from build123d import *

# Parameters (mm, degrees)
CUT_EXTRUDE1_DEPTH      = 874.621652083
CUT_EXTRUDE1_DEPTH_BACK = 874.621652083
SKETCH6_R               = 38.1
SKETCH9_W               = 1605.930086896
SKETCH9_H               = 1331.723127606
CUT_EXTRUDE8_DEPTH      = 762.168569892


with BuildPart() as part:
    # Sketch4 → Revolve3 (revolve)
    with BuildSketch(Plane.XY, mode=Mode.PRIVATE) as revolve3_sk:
        with BuildLine():
            Line((25.4, 650.00817936), (25.4, 83.643188795))
            ThreePointArc((25.4, 83.643188795), (205.276173143, 67.197534451), (381, 25.4))
            Line((381, 25.4), (412.7373, 25.4))
            Line((412.7373, 25.4), (412.7373, 488.95))
            Line((412.7373, 488.95), (411.1498, 488.95))
            Line((411.1498, 488.95), (411.1498, 514.35))
            ThreePointArc((411.1498, 514.35), (404.683813004, 537.626492136), (387.141395745, 554.23575674))
            ThreePointArc((387.141395745, 554.23575674), (211.762891066, 622.866495309), (25.4, 650.00817936))
        make_face()
    revolve(revolve3_sk.sketch.rotate(Axis((0, 588.703209944, 0), (0, -1, 0)), 90), axis=Axis((0, 588.703209944, 0), (0, -1, 0)))

    # Sketch6 → Cut-Extrude1 (cut, two sides: drawn at the far end of the back side and taken through both)
    with BuildSketch(Plane(origin=(0, 0, 0), x_dir=(1, 0, 0), z_dir=(0, 1, 0)).offset(-CUT_EXTRUDE1_DEPTH_BACK)):
        with Locations(Location((143.684097937, 143.684097937, 0), (0, 0, 131.539783137))):
            Circle(SKETCH6_R)
        with Locations(Location((-85.876030786, 184.161742326, 0), (0, 0, 134.878306021))):
            Circle(SKETCH6_R)
        with Locations(Location((-85.876030786, -184.161742326, 0), (0, 0, 134.996806388))):
            Circle(SKETCH6_R)
        with Locations(Location((143.684097937, -143.684097937, 0), (0, 0, 135))):
            Circle(SKETCH6_R)
    extrude(amount=CUT_EXTRUDE1_DEPTH + CUT_EXTRUDE1_DEPTH_BACK, mode=Mode.SUBTRACT)

    # Sketch9 → Cut-Extrude8 (cut, through all)
    with BuildSketch(Plane(origin=(-95.081116315, 261.233220092, 0), x_dir=(-0.9396926207859104, -0.34202014332566316, 0), z_dir=(0.34202014332566316, -0.9396926207859104, 0))):
        Rectangle(SKETCH9_W, SKETCH9_H)
    extrude(amount=-CUT_EXTRUDE8_DEPTH, mode=Mode.SUBTRACT)


solid = part.part
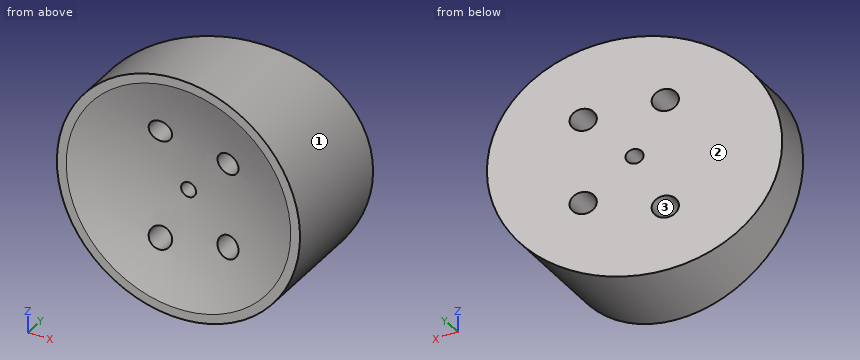
Model file for the job. Use its own axes, mm. Face numbers are marked on the shaded views. Give positions to 0.01 mm unless a question says otherwise; leave off trailing zeros. Order: outer loops, then holes, each group sorted by start corner. A loop starts at its lowest first (then second) coordinate and runs counter-clockwise, first axis right, second up. Notation, with made-up numbers: (14, -1) - (18, -1) arc R15 cw to (18, 3) - close; hole circle Ø3 at (42, 79.25). An arc over 180 degrees is marked (long way). One line per item, written item: value.
Item 1: Slice it at D-D (x = 292). List the corners of the cut face in (y, z), then the cut area to 3 significant figures.
Response values:
outline: (25.4, -291.7) - (402.12, -291.7) - (402.12, 291.7) - (25.4, 291.7) - (25.4, 244.74) arc R1235.98 cw to (25.4, -244.74) - close
area: 212,000 mm2
Item 2: Two-plate mould, pull along Z, no slides. Class the marked faces 1, 2 and 3: released by +Z, released by -Z, zero draft, split by the parting line, or undercut.
Response values:
face 1: split by the parting line
face 2: zero draft
face 3: undercut
Item 3: Slice it at B-B (x = 0). List the corners of the cut face in (y, z).
Response values:
outline: (25.4, -412.74) - (295.84, -412.74) - (295.84, -25.4) - (83.64, -25.4) arc R1270 cw to (25.4, -381) - close; (25.4, 381) arc R1270 cw to (83.64, 25.4) - (295.84, 25.4) - (295.84, 412.74) - (25.4, 412.74) - close
Item 4: Wall check: line 1 (Z direction, x = 156, y = 281.5); line 2 (Z direction, x = 115.5, y = 288); line 3 (X direction, y = 153.5, z = -300.5). Give the ranges that are in metal, low to high.
Response values:
line 1: -382.12 to -179.74, -107.63 to 107.63, 179.74 to 382.12
line 2: -396.25 to -169.32, -118.05 to 118.05, 169.32 to 396.25
line 3: -282.93 to 282.93
Item 5: Slice it at A-A (z = 0). List the corners of the cut face in (x, y), then the cut area to 3 significant figures.
Response values:
outline: (-412.74, 25.4) - (-381, 25.4) arc R1270 cw to (-25.4, 83.64) - (-25.4, 286.6) - (-412.74, 145.62) - close; (25.4, 83.64) arc R1270 cw to (381, 25.4) - (412.74, 25.4) - (412.74, 446.06) - (25.4, 305.08) - close
area: 183,000 mm2
Item 6: Pin check, flat tips, straight feed: pin 1 Ø2 at (y, z) = (123, 55.5) entering from +X; pin 2 Ø6 at (y, z) = (134, 166) entering from -X; pin 3 Ø12 at (x, z) = (-7, -241) entering from +Y. Stop position of each tip, or through.
Response values:
pin 1: x = 409.12
pin 2: x = -379.19
pin 3: y = 295.48
Item 7: Slice it at C-C (y = 229). List the corners of the cut face in (x, z).
Response values:
outline: (-183.64, -369.63) arc R412.74 ccw (long way) to (-183.64, 369.63) - close; hole circle Ø76.2 at (-85.88, -184.16); hole circle Ø76.2 at (-85.88, 184.16); hole circle Ø50.8 at (0, 0); hole circle Ø76.2 at (143.68, -143.68); hole circle Ø76.2 at (143.68, 143.68)
